```python
from build123d import *

# Parameters (mm, degrees)
SKETCH1_R            = 29.705
BASE_DEPTH           = 12
SUPPORT_SHAPE_DEPTH  = 30
SKETCH3_R            = 4.8
PEN_HOLE_DEPTH       = 86.315453863
SKETCH5_R            = 2
BOLT_HOLES_DEPTH     = 86.315453863
ELASTIC_HOLES_REACH  = 68.458
SKETCH8_R            = 4
DECORATIVE_FILLET_R  = 8
SKETCH9_W            = 13.029443146
SKETCH9_H            = 56.051778338
SKETCH9_W_2          = 11.207609874
SKETCH9_H_2          = 62.108426406
DECORATIVE_CUT_DEPTH = 81.091988787


with BuildPart() as part:
    # Sketch1 → Base (new body)
    with BuildSketch(Plane(origin=(0, 6, 0), x_dir=(1, 0, 0), z_dir=(0, 1, 0))):
        with Locations(Location((1.546657586, 37.660128709, 0), (0, 0, 270))):
            Circle(SKETCH1_R)
    extrude(amount=BASE_DEPTH)

    # Sketch2 → Support Shape (add)
    with BuildSketch(Plane(origin=(0, 18, 0), x_dir=(1, 0, 0), z_dir=(0, 1, 0))):
        with BuildLine():
            Line((-7.618493804, 41.660128709), (-23.453342414, 41.660128709))
            Line((-23.453342414, 41.660128709), (-23.453342414, 33.660128709))
            Line((-23.453342414, 33.660128709), (-7.618493804, 33.660128709))
            ThreePointArc((-7.618493804, 33.660128709), (-8.453342414, 37.660128709), (-7.618493804, 41.660128709))
        make_face()
        with BuildLine():
            ThreePointArc((10.711808976, 41.660128709), (1.546657586, 47.660128709), (-7.618493804, 41.660128709))
            Line((-7.618493804, 41.660128709), (10.711808976, 41.660128709))
        make_face()
        with BuildLine():
            Line((10.711808976, 41.660128709), (-7.618493804, 41.660128709))
            ThreePointArc((-7.618493804, 41.660128709), (-8.453342414, 37.660128709), (-7.618493804, 33.660128709))
            Line((-7.618493804, 33.660128709), (10.711808976, 33.660128709))
            ThreePointArc((10.711808976, 33.660128709), (11.335720716, 35.617032272), (11.546657586, 37.660128709))
            ThreePointArc((11.546657586, 37.660128709), (11.335720716, 39.703225146), (10.711808976, 41.660128709))
        make_face()
        with BuildLine():
            Line((10.711808976, 33.660128709), (-7.618493804, 33.660128709))
            ThreePointArc((-7.618493804, 33.660128709), (1.546657586, 27.660128709), (10.711808976, 33.660128709))
        make_face()
        with BuildLine():
            Line((26.546657586, 41.660128709), (10.711808976, 41.660128709))
            ThreePointArc((10.711808976, 41.660128709), (11.335720716, 39.703225146), (11.546657586, 37.660128709))
            ThreePointArc((11.546657586, 37.660128709), (11.335720716, 35.617032272), (10.711808976, 33.660128709))
            Line((10.711808976, 33.660128709), (26.546657586, 33.660128709))
            Line((26.546657586, 33.660128709), (26.546657586, 41.660128709))
        make_face()
    extrude(amount=SUPPORT_SHAPE_DEPTH)

    # Sketch3 → Pen Hole (cut, through all)
    with BuildSketch(Plane(origin=(0, 48, 0), x_dir=(1, 0, 0), z_dir=(0, 1, 0))):
        with Locations(Location((1.546657586, 37.660128709, 0), (0, 0, 270))):
            Circle(SKETCH3_R)
    extrude(amount=-PEN_HOLE_DEPTH, mode=Mode.SUBTRACT)

    # Sketch5 → Bolt Holes (cut, through all)
    with BuildSketch(Plane.XZ.offset(-6)):
        with Locations(Location((-7.953342414, -14.026565813, 0), (0, 0, 270))):
            Circle(SKETCH5_R)
        with Locations(Location((1.546657586, -12.410128709, 0), (0, 0, 270))):
            Circle(SKETCH5_R)
        with Locations(Location((11.046657586, -14.026565813, 0), (0, 0, 270))):
            Circle(SKETCH5_R)
        with Locations(Location((11.046657586, -60.376565813, 0), (0, 0, 270))):
            Circle(SKETCH5_R)
        with Locations(Location((1.546657586, -62.910128709, 0), (0, 0, 270))):
            Circle(SKETCH5_R)
        with Locations(Location((-7.953342414, -60.376565813, 0), (0, 0, 270))):
            Circle(SKETCH5_R)
    extrude(amount=-BOLT_HOLES_DEPTH, mode=Mode.SUBTRACT)

    # Sketch8 → Elastic Holes (cut, up to next)
    with BuildSketch(Plane.XY.offset(-33.660128709), mode=Mode.PRIVATE) as elastic_holes_sk1:
        with Locations((18.629233281, 40)):
            Circle(SKETCH8_R)
    elastic_holes_tool1 = extrude(elastic_holes_sk1.sketch, amount=-ELASTIC_HOLES_REACH, mode=Mode.PRIVATE) & part.part
    # Sketch8 → Elastic Holes (cut, up to next)
    with BuildSketch(Plane.XY.offset(-33.660128709), mode=Mode.PRIVATE) as elastic_holes_sk2:
        with Locations(Location((-15.535918109, 40, 0), (0, 0, 180))):
            Circle(SKETCH8_R)
    elastic_holes_tool2 = extrude(elastic_holes_sk2.sketch, amount=-ELASTIC_HOLES_REACH, mode=Mode.PRIVATE) & part.part
    add(elastic_holes_tool1.solids().sort_by_distance((18.629233, 40, -33.660129))[0], mode=Mode.SUBTRACT)
    add(elastic_holes_tool2.solids().sort_by_distance((-15.535918, 40, -33.660129))[0], mode=Mode.SUBTRACT)

    # Decorative Fillet
    decorative_fillet_edges = [part.edges().sort_by_distance(p)[0] for p in [
        (26.546657586, 48, -37.660128709),
        (-23.453342414, 48, -37.660128709),
    ]]
    fillet(decorative_fillet_edges, radius=DECORATIVE_FILLET_R)

    # Sketch9 → Decorative Cut (cut, through all)
    with BuildSketch(Plane(origin=(0, 18, 0), x_dir=(1, 0, 0), z_dir=(0, 1, 0))):
        with Locations((33.061379159, 37.205930485)):
            Rectangle(SKETCH9_W, SKETCH9_H)
        with Locations((-29.057147351, 40.234254519)):
            Rectangle(SKETCH9_W_2, SKETCH9_H_2)
    extrude(amount=-DECORATIVE_CUT_DEPTH, mode=Mode.SUBTRACT)


solid = part.part
```
The listing builds one solid part. Answer for the finished solid, in the listing's coordinates (mm). A direction names the side the tool comes from. Coordinates: 2 decimals unless noted, no trailing zeros. Loops run counter-clockwise (first coordinate to the right, second up) from the corner with the lowest first, then second, coordinate; pieces in that order, holes last. Notation, with made-up numbers: (-34, 48) -> (2, 48) arc R25 cw to (2, 80) -> close; hole circle Ø7 at (32.5, 76). An arc over 180 degrees is marked (long way). Return JSON: item names as keys, results as strings. Group by question number.
(1) A cutting plane is placed at B-B on y = 12. Write down the section's boundary in (x, z) (3 decimals).
(2) Which of the six approach directions +Z, -Z, +X, -X, +Y, -Y give full straight-line access (tool end or side, diameter ignored) to faces 5 (the flat face through (-16, 33, -33.66)), 6 (the flat face through (-15, 33, -41.66)), 7 (the flat face through (19, 33, -33.66)), 8 (the cylindrical face through (1.71, 32.79, -47.66))?
(3) A cutting plane is placed at D-D on y = 42.5. Write down the section's boundary in (x, z).
(4) Find the intervals of material crossed by probe 1 along Z at (x, y) = (1.5, 16); probe 2 along Y at (x, z) = (21, -43.5); probe 3 along X at (y, z) = (11, -37.5), in increasing order. Write a range as from..to.
(5) A cutting plane is placed at A-A on z = -37. Write down the section's boundary in (x, y).
(6) A cutting plane is placed at C-C on x = -2. Write down the section's boundary in (y, z), and give its area (3 significant figures).
(7) Given pin 1 Ø4.5 at (x, z) = (11.05, -14.03) entering from +Y; pin 2 Ø6 at (x, y) = (-15.5, 38.5) entering from +Z; pin 3 Ø8 at (x, y) = (-16, 29.5) entering from -Z, each flat-ended and moving along its own axis, determine where each tip first touches the part or whether it passes through.
(8) Determine the mould class of faces 1 (the cylindrical face through (24.27, 45.59, -37.72)), 2 (the flat face through (-23.453, 19, -38)), 3 (the flat face through (19, 33, -41.66)), 4 (the cylindrical face through (-15.015, 36.034, -37.604)) for opening direction X: released by +X, released by -X, zero draft, split by the parting line, or undercut.
The answers:
{
 "1": {"outline": "(-23.453, -53.703) arc R29.705 ccw to (26.547, -53.703) -> (26.547, -21.617) arc R29.705 ccw to (-23.453, -21.617) -> close; hole circle Ø4 at (-7.953, -60.377); hole circle Ø4 at (-7.953, -14.027); hole circle Ø9.6 at (1.547, -37.66); hole circle Ø4 at (1.547, -62.91); hole circle Ø4 at (1.547, -12.41); hole circle Ø4 at (11.047, -60.377); hole circle Ø4 at (11.047, -14.027)"},
 "2": {"face 5": "+Z, -X, +Y", "face 6": "-Z, -X, +Y", "face 7": "+Z, +X, +Y", "face 8": "-Z, +Y"},
 "3": {"outline": "(-23.05, -41.66) -> (-18.66, -41.66) -> (-18.66, -33.66) -> (-23.05, -33.66) -> close; (-12.41, -41.66) -> (-7.62, -41.66) arc R10 ccw to (10.71, -41.66) -> (15.51, -41.66) -> (15.51, -33.66) -> (10.71, -33.66) arc R10 ccw to (-7.62, -33.66) -> (-12.41, -33.66) -> close; (21.75, -41.66) -> (26.15, -41.66) -> (26.15, -33.66) -> (21.75, -33.66) -> close; hole circle Ø9.6 at (1.55, -37.66)"},
 "4": {"probe 1": "z = -67.37..-64.91, -60.91..-42.46, -32.86..-14.41, -10.41..-7.96", "probe 2": "y = 6..18", "probe 3": "x = -23.45..-3.25, 6.34..26.55"},
 "5": {"outline": "(-23.45, 6) -> (-3.21, 6) -> (-3.21, 48) -> (-15.45, 48) arc R8 ccw to (-23.45, 40) -> close; (6.3, 6) -> (26.55, 6) -> (26.55, 40) arc R8 ccw to (18.55, 48) -> (6.3, 48) -> close; hole circle Ø8 at (-15.54, 40); hole circle Ø8 at (18.63, 40)"},
 "6": {"outline": "(6, -67.15) -> (18, -67.15) -> (18, -47.01) -> (48, -47.01) -> (48, -40.89) -> (6, -40.89) -> close; (6, -34.43) -> (48, -34.43) -> (48, -28.31) -> (18, -28.31) -> (18, -8.17) -> (6, -8.17) -> close", "area": "997 mm^2"},
 "7": {"pin 1": "stops at y = 18", "pin 2": "stops at z = -33.66", "pin 3": "stops at z = -41.66"},
 "8": {"face 1": "released by +X", "face 2": "released by -X", "face 3": "zero draft", "face 4": "undercut"}
}
